Source: CAD feature listing. Evaluate the final solid. Frame: model axes, mm. Face numbers are marked on the shaded views. A direction names the side the tool comes from. Round coordinates to 2 decimals unless told otherwise and drop trailing zeros. Order: outer loops, then holes, each group sorted by start corner. A loop starts at its lowest first (then second) coordinate and runs counter-clockwise, first axis right, second up. Notation, with made-up numbers: (68, 65.5) - (93, 65.5) arc R13 cw to (93, 79.5) - close; hole circle Ø3 at (58, -33.5). An arc over 180 degrees is marked (long way). Put each result on its own line as item: value. Start each with the question number.
1) Section A-A on z = 10.16. Output: boundary loops of the cut face in (x, y) (3 decimals), then the cut area to 3 significant figures.
2) Section C-C on x = 6.25. Output: boundary loops of the cut face in (y, z).
3) Mould query, pull axis Z, two halves, no side actions, for the marked faces 4, 5, 6 and 7. Classes: +Z half, -Z half, draft (parallel to the pull), parting line (faces both ways), or undercut.
4) Access query for the marked faces 1, 2 and 3. Directions: +Z, -Z, +X, -X, +Y, -Y. A direction counts if a zero-diameter tool reaches every point of the face in a straight line with its end or side. Return the directions, or none.
5) Line query: probe 1 along X at (y, z) = (17, 3.75); probe 2 along Y at (x, z) = (5.5, 10.16); probe 3 along Z at (x, y) = (9.25, 10). Output: solid intervals per line, ascending. Write a range as [from, to].
6) Section D-D on y = 18. Output: boundary loops of the cut face in (x, z), then the cut area to 3 significant figures.
7) Contact query for flat-ended pins moving along their axis: P1, Ø1.5, axis at x = 3.5, y = 16, coming from the +Z side; P2, Ø4, axis at x = 11.5, y = 4, coming from the -Z side; P3, Ø5, axis at x = 16.5, z = 5.5, coming from the -Y side; P4, Ø5, axis at x = -1, z = 7, coming from the +Y side. Output: stop coordinate, or through.
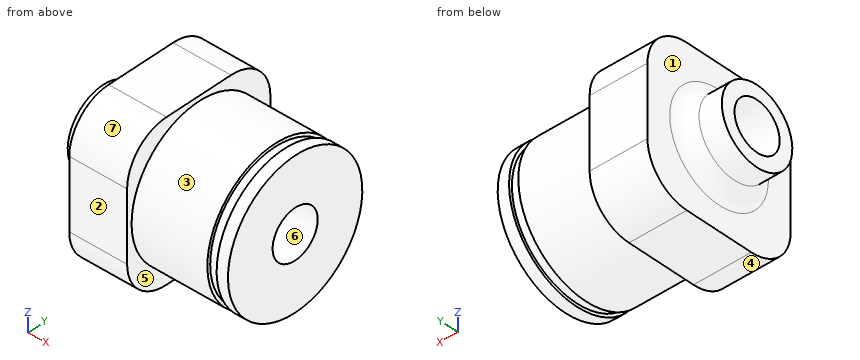
Autodesk Inventor part; units mm, degrees
ref_plane "YZ Plane" through (0, 0, 0) normal (1, 0, 0) x (0, 1, 0)
ref_plane "XZ Plane" through (0, 0, 0) normal (0, 1, 0) x (-1, 0, 0)
ref_plane "XY Plane" through (0, 0, 0) normal (0, 0, 1) x (1, 0, 0)
sketch "Sketch1" plane through (0, 0, 0) normal (1, 0, 0) x (0, 1, 0)
  line L0 (0, 0) -> (20.32, 0)
  line L1 (20.32, 0) -> (20.32, 20.32)
  line L2 (20.32, 20.32) -> (0, 20.32)
  line L3 (0, 20.32) -> (0, 0)
  dimension "d0" = 20.32
  dimension "d1" = 20.32
extrude "Extrusion1" add sketch "Sketch1" along normal blind 7.62
sketch "Sketch2" plane through (7.62, 0, 0) normal (1, 0, 0) x (0, 0, -1)
  circle A0 centre (-10.16, 10.16) radius 9.525
  point P0 (0, 0)
  dimension "d4" = 19.05
extrude "Extrusion2" add sketch "Sketch2" along normal blind 12.7
fillet "Fillet1" radius 5.588 4 edges at (3.81, 20.32, 0) (3.81, 0, 0) (3.81, 0, 20.32) (3.81, 20.32, 20.32)
sketch "Sketch3" plane through (20.32, 10.16, 10.16) normal (1, 0, 0) x (0, 0, -1)
  circle A0 centre (0, 0) radius 9.525
  circle A1 centre (0, 0) radius 9.125
  point P0 (10.16, -10.16)
  dimension "d8" = 18.25
extrude "Extrusion3" cut sketch "Sketch3" against normal blind 2.72
sketch "Sketch4" plane through (20.32, 10.16, 10.16) normal (1, 0, 0) x (0, 0, -1)
  circle A0 centre (0, 0) radius 9.525
  point P0 (10.16, -10.16)
extrude "Extrusion4" add sketch "Sketch4" against normal blind 1.5
sketch "Sketch5" plane through (0, 0, 0) normal (-1, 0, 0) x (0, 0, 1)
  circle A0 centre (10.16, 10.16) radius 9.125
  circle A1 centre (10.16, 10.16) radius 4
  point P0 (0, 0)
  dimension "d13" = 8
extrude "Extrusion5" cut sketch "Sketch5" against normal blind 25 contours A1
sketch "Sketch6" plane through (0, 0, 0) normal (-1, 0, 0) x (0, 0, 1)
  circle A0 centre (10.16, 10.16) radius 4
  circle A1 centre (10.16, 10.16) radius 4
  circle A2 centre (10.16, 10.16) radius 5
  point P0 (0, 0)
  dimension "d16" = 10
extrude "Extrusion6" add sketch "Sketch6" along normal blind 5
fillet "Fillet2" radius 2 1 edges at (0, 10.16, 5.16)
sketch "Sketch7" plane through (20.32, 10.16, 10.16) normal (1, 0, 0) x (0, 0, -1)
  circle A0 centre (0, 0) radius 4
  circle A1 centre (0, 0) radius 4
  circle A2 centre (0, 0) radius 3.2
  point P0 (10.16, -10.16)
  dimension "d20" = 6.4
extrude "Extrusion7" add sketch "Sketch7" against normal blind 25.32
properties part number "_3DPrint"
Answer sheet:
1. outline: (-5, 5.16) - (-2, 5.16) arc R2 cw to (0, 3.16) - (0, 0) - (7.62, 0) - (7.62, 0.635) - (17.6, 0.635) - (17.6, 1.035) - (18.82, 1.035) - (18.82, 0.635) - (20.32, 0.635) - (20.32, 6.96) - (-5, 6.96) - close; (-5, 13.36) - (20.32, 13.36) - (20.32, 19.685) - (18.82, 19.685) - (18.82, 19.285) - (17.6, 19.285) - (17.6, 19.685) - (7.62, 19.685) - (7.62, 20.32) - (0, 20.32) - (0, 17.16) arc R2 cw to (-2, 15.16) - (-5, 15.16) - close
1. area: 285 mm^2
2. outline: (0, 5.59) arc R5.59 ccw to (5.59, 0) - (14.73, 0) arc R5.59 ccw to (20.32, 5.59) - (20.32, 14.73) arc R5.59 ccw to (14.73, 20.32) - (5.59, 20.32) arc R5.59 ccw to (0, 14.73) - close; hole circle Ø6.4 at (10.16, 10.16)
3. face 4: -Z half
3. face 5: draft
3. face 6: undercut
3. face 7: +Z half
4. face 1: -X
4. face 2: +Z, -Z, +X, -X, -Y
4. face 3: +X
5. probe 1: [0, 17.6], [18.82, 20.32]
5. probe 2: [0, 6.96], [13.36, 20.32]
5. probe 3: [0.64, 6.96], [13.36, 19.68]
6. outline: (0, 1.06) - (7.62, 1.06) - (7.62, 4.75) - (17.6, 4.75) - (17.6, 5.49) - (18.82, 5.49) - (18.82, 4.75) - (20.32, 4.75) - (20.32, 15.57) - (18.82, 15.57) - (18.82, 14.83) - (17.6, 14.83) - (17.6, 15.57) - (7.62, 15.57) - (7.62, 19.26) - (0, 19.26) - close
6. area: 274 mm^2
7. P1: z = 20.3
7. P2: z = 1.59
7. P3: y = 0.88
7. P4: y = 20.32
